Check sheet for the modelled part. Datum: model origin and axes. Units: mm. Face numbers are marked on the shaded views. A direction names the side the tool comes from. Coordinates: 2 decimals unless noted, no trailing zeros. Loops run counter-clockwise (first coordinate to the right, second up) from the corner with the lowest first, then second, coordinate; pieces in that order, holes last. Notation, with made-up numbers: (38.5, 8) - (80.5, 8) arc R26 ccw to (80.5, 27) - close; hole circle Ø5 at (-17, -27.75). An arc over 180 degrees is marked (long way). Write each question's results on one line, items separated by ' | '. Start each with the question number.
1. Cross-section at C-C (z = 35). Record the cut outline in (x, y), and give its area (3 significant figures).
2. Cross-section at D-D (x = 0). Record the cut outline in (y, z).
3. Draft check along X on the marked faces 1, 2 and 3. Enter one of: released by +X, released by -X, zero draft, split by the parting line, or undercut.
4. Thickness scan on line 1 (Y direction, x = 2.25, z = 22); line 2 (X direction, y = -9.25, z = 35). Record the ranges inside material, lowest first. Write a range as [from, to].
5. Cross-section at A-A (y = -1.5). Record the cut outline in (x, z), and give its area (3 significant figures).
6. Tool access check on the marked faces 4 and 5. Record the directions out of +Z, -Z, +X, -X, +Y, -Y that give a thin tool (end or side, any length) a straight path to the whole face; none if there is none.
7. Gauge pin test, flat ends, axial feed: P1, Ø4.5, axis at x = 0, z = 10, coming from the -Y side; P2, Ø2.5, axis at x = 0, z = 10, coming from the +Y side. Record the tip position at first contact, or that the pin passes through.
```python
from build123d import *

# Parameters (mm, degrees)
SKETCH_1_W          = 20
SKETCH_1_H          = 20
SKETCH_1_W_2        = 18
SKETCH_1_H_2        = 18
EXTRUDE_1_DEPTH     = 45
CUT_EXTRUDE_1_REACH = 52.249
SKETCH_2_R          = 2


with BuildPart() as part:
    # 草图1 → 凸台-拉伸1 (new body)
    with BuildSketch(Plane.XY):
        Rectangle(SKETCH_1_W, SKETCH_1_H)
        Rectangle(SKETCH_1_W_2, SKETCH_1_H_2, mode=Mode.SUBTRACT)
    extrude(amount=EXTRUDE_1_DEPTH)

    # 切除-拉伸1: up to this face of the body (flat: up to its plane)
    cut_extrude_1_end = Plane(part.part.faces().sort_by_distance((0, -10, 22.5))[0])
    # 草图2 → 切除-拉伸1 (cut, up to the picked face)
    with BuildSketch(Plane(origin=(0, 10, 0), x_dir=(1, 0, 0), z_dir=(0, 1, 0)), mode=Mode.PRIVATE) as cut_extrude_1_sk1:
        with Locations(Location((0, -10, 0), (0, 0, 270))):
            Circle(SKETCH_2_R)
    cut_extrude_1_tool1 = split(extrude(cut_extrude_1_sk1.sketch, amount=-CUT_EXTRUDE_1_REACH, mode=Mode.PRIVATE), bisect_by=cut_extrude_1_end, keep=Keep.BOTH, mode=Mode.PRIVATE)
    # 草图2 → 切除-拉伸1 (cut, up to the picked face)
    with BuildSketch(Plane(origin=(0, 10, 0), x_dir=(1, 0, 0), z_dir=(0, 1, 0)), mode=Mode.PRIVATE) as cut_extrude_1_sk2:
        with Locations(Location((0, -35, 0), (0, 0, 270))):
            Circle(SKETCH_2_R)
    cut_extrude_1_tool2 = split(extrude(cut_extrude_1_sk2.sketch, amount=-CUT_EXTRUDE_1_REACH, mode=Mode.PRIVATE), bisect_by=cut_extrude_1_end, keep=Keep.BOTH, mode=Mode.PRIVATE)
    add(cut_extrude_1_tool1.solids().sort_by(Axis((0, 10, 10), (0, -1, 0)))[0], mode=Mode.SUBTRACT)
    add(cut_extrude_1_tool2.solids().sort_by(Axis((0, 10, 35), (0, -1, 0)))[0], mode=Mode.SUBTRACT)


solid = part.part
```
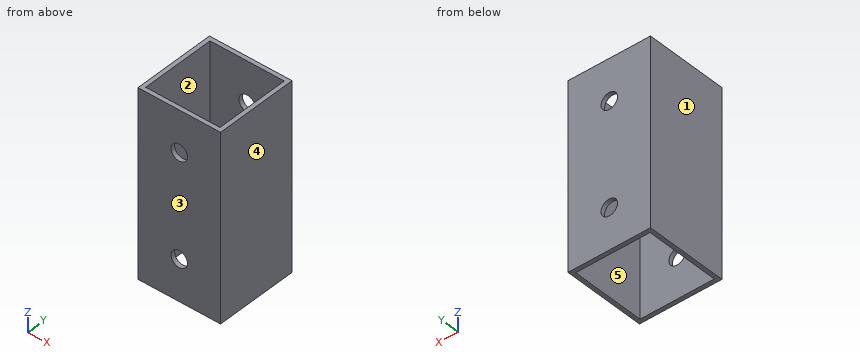
Established:
1) outline: (-10, -10) - (-2, -10) - (-2, -9) - (-9, -9) - (-9, 9) - (-2, 9) - (-2, 10) - (-10, 10) - close; (2, -10) - (10, -10) - (10, 10) - (2, 10) - (2, 9) - (9, 9) - (9, -9) - (2, -9) - close | area: 68.0 mm^2
2) outline: (-10, 0) - (-9, 0) - (-9, 8) - (-10, 8) - close; (-10, 12) - (-9, 12) - (-9, 33) - (-10, 33) - close; (-10, 37) - (-9, 37) - (-9, 45) - (-10, 45) - close; (9, 0) - (10, 0) - (10, 8) - (9, 8) - close; (9, 12) - (10, 12) - (10, 33) - (9, 33) - close; (9, 37) - (10, 37) - (10, 45) - (9, 45) - close
3) face 1: released by -X | face 2: undercut | face 3: zero draft
4) line 1: [-10, -9], [9, 10] | line 2: [-10, -2], [2, 10]
5) outline: (-10, 0) - (-9, 0) - (-9, 45) - (-10, 45) - close; (9, 0) - (10, 0) - (10, 45) - (9, 45) - close | area: 90.0 mm^2
6) face 4: +Z, -Z, +X, +Y, -Y | face 5: +Z, -Z
7) P1: y = -10 | P2: through
